```python
from build123d import *

# Parameters (mm, degrees)
F1_DEPTH = 19.05
F2_DEPTH = 31.75


with BuildPart() as f1:
    # F0 (on Front) → F1 (new body)
    with BuildSketch(Plane.XZ):
        with BuildLine():
            ThreePointArc((-18.047368, 41.993555), (-24.667298, 21.714159), (-26.906852, 0.4995))
            Line((-26.906852, 0.4995), (28.711593, 0.4995))
            ThreePointArc((28.711593, 0.4995), (26.472039, 21.714159), (19.852109, 41.993555))
            ThreePointArc((19.852109, 41.993555), (0.902371, 47.536649), (-18.047368, 41.993555))
        make_face()
    extrude(amount=F1_DEPTH)

    # F0 (on Front) → F2 (join)
    with BuildSketch(Plane.XZ):
        with BuildLine():
            ThreePointArc((-26.906852, -42.446553), (-25.04698, -46.936681), (-20.556852, -48.796553))
            Line((-20.556852, -48.796553), (22.361593, -48.796553))
            ThreePointArc((22.361593, -48.796553), (26.851721, -46.936681), (28.711593, -42.446553))
            Line((28.711593, -42.446553), (28.711593, 0.4995))
            Line((28.711593, 0.4995), (-26.906852, 0.4995))
            Line((-26.906852, 0.4995), (-26.906852, -42.446553))
        make_face()
    extrude(amount=F2_DEPTH)


solid = f1.part
```
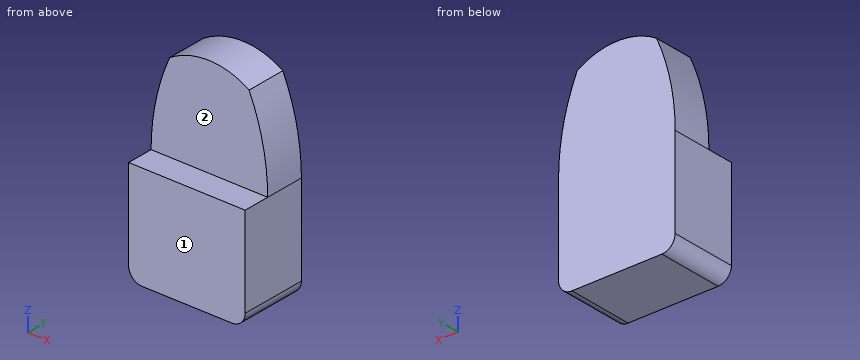
CAD build for the part. Positions are in the model's coordinates, mm. Face numbers are marked on the shaded views. A direction names the side the tool comes from. Round coordinates to 2 decimals unless told otherwise and drop trailing zeros. Order: outer loops, then holes, each group sorted by start corner. A loop starts at its lowest first (then second) coordinate and runs counter-clockwise, first axis right, second up.
Item 1: Tool access for the marked faces 1 and 2: list every direction of +Z, -Z, +X, -X, +Y, -Y with a clear straight run to the whole face (end or side of a thin tool).
Item 2: Saw through at A-A on y = -12. Write the cut outline in (x, z), then the cut area to 3 significant figures.
Item 3: Saw through at D-D on z = 30. Write the cut outline in (x, y), then the cut area to 3 significant figures.
Item 4: Saw through at C-C on y = -22. Write the cut outline in (x, z).
Item 5: Saw through at B-B on x = -14. Write the cut outline in (y, z), then the cut area to 3 significant figures.
Item 6: Pin check, flat tips, straight feed: pin 1 (6.5 mm diameter, centred on x = 0, y = -28.5, fed in from +Z); pin 2 (1.5 mm diameter, centred on x = -7, y = -17, fed in from +Z); pin 3 (3 mm diameter, centred on y = -20, z = 15, fed in from -X). Stop position of each tip, or through.
Item 7: Probe line 1 along Z through (x, y) = (8, -25); line 2 along Y through (x, z) = (21.5, 26); line 3 along X through (y, z) = (-16.5, 42). List the from-to ranges inside material, lowest first.
Reported:
1. face 1: +Z, -Z, +X, -X, -Y
1. face 2: +Z, +X, -X, -Y
2. outline: (-26.91, -42.45) arc R6.35 ccw to (-20.56, -48.8) - (22.36, -48.8) arc R6.35 ccw to (28.71, -42.45) - (28.71, 0.5) arc R101.6 ccw to (19.85, 41.99) arc R35.16 ccw to (-18.05, 41.99) arc R101.6 ccw to (-26.91, 0.5) - close
2. area: 4,930 mm2
3. outline: (-22.53, -19.05) - (24.33, -19.05) - (24.33, 0) - (-22.53, 0) - close
3. area: 893 mm2
4. outline: (-26.91, -42.45) arc R6.35 ccw to (-20.56, -48.8) - (22.36, -48.8) arc R6.35 ccw to (28.71, -42.45) - (28.71, 0.5) - (-26.91, 0.5) - close
5. outline: (-31.75, -48.8) - (0, -48.8) - (0, 44.22) - (-19.05, 44.22) - (-19.05, 0.5) - (-31.75, 0.5) - close
5. area: 2,400 mm2
6. pin 1: stops at z = 0.5
6. pin 2: stops at z = 46.8
6. pin 3: stops at x = -26.03
7. line 1: z = -48.8 to 0.5
7. line 2: y = -19.05 to 0
7. line 3: x = -18.04 to 19.84
